from build123d import *
from build123d.topology import SkipClean

# Parameters (mm, degrees)
SKETCH1_R           = 18.161
BOSS_EXTRUDE1_DEPTH = 1.651
BOSS_EXTRUDE2_DEPTH = 5.8928
CUT_EXTRUDE1_REACH  = 45.689
SKETCH5_R           = 13.462
BOSS_EXTRUDE3_DEPTH = 13.335
SKETCH6_R           = 13.462
BOSS_EXTRUDE4_DEPTH = 9.652
BOSS_EXTRUDE4_TAPER = 4
SKETCH7_R           = 13.462
BOSS_EXTRUDE5_DEPTH = 15.24
SKETCH8_R           = 9.398
CUT_EXTRUDE3_DEPTH  = 63.427016824


with BuildPart() as part:
    # Sketch1 → Boss-Extrude1 (new body)
    with BuildSketch(Plane(origin=(0, 0, 0), x_dir=(1, 0, 0), z_dir=(0, 1, 0))):
        with Locations(Location((-14.328841802, 9.162551515, 0), (0, 0, 90))):
            Circle(SKETCH1_R)
    extrude(amount=BOSS_EXTRUDE1_DEPTH)

    # Sketch2 → Boss-Extrude2 (add)
    with BuildSketch(Plane(origin=(0, 1.651, 0), x_dir=(1, 0, 0), z_dir=(0, 1, 0))):
        Polygon((2.466775283, 0.14327327), (1.879890825, 19.198343461), (-14.91572626, 28.217621706), (-31.124458887, 18.18182976), (-30.537574428, -0.87324043), (-13.741957343, -9.892518675), align=None)
    extrude(amount=BOSS_EXTRUDE2_DEPTH)

    # Sketch3 → Cut-Extrude1 (cut, up to next)
    with BuildSketch(Plane(origin=(0, 7.5438, 0), x_dir=(1, 0, 0), z_dir=(0, 1, 0)), mode=Mode.PRIVATE) as cut_extrude1_sk1:
        with BuildLine():
            Line((-13.183471606, 27.287397669), (-14.91572626, 28.217621706))
            Line((-14.91572626, 28.217621706), (-16.587451234, 27.182557187))
            ThreePointArc((-16.587451234, 27.182557187), (-14.887924337, 27.314943857), (-13.183471606, 27.287397669))
        make_face()
    cut_extrude1_tool1 = extrude(cut_extrude1_sk1.sketch, amount=-CUT_EXTRUDE1_REACH, mode=Mode.PRIVATE) & part.part
    # Sketch3 → Cut-Extrude1 (cut, up to next)
    with BuildSketch(Plane(origin=(0, 7.5438, 0), x_dir=(1, 0, 0), z_dir=(0, 1, 0)), mode=Mode.PRIVATE) as cut_extrude1_sk2:
        with BuildLine():
            Line((1.879890825, 19.198343461), (0.147636171, 20.128567497))
            ThreePointArc((0.147636171, 20.128567497), (1.112049838, 18.722927364), (1.940420505, 17.233054906))
            Line((1.940420505, 17.233054906), (1.879890825, 19.198343461))
        make_face()
    cut_extrude1_tool2 = extrude(cut_extrude1_sk2.sketch, amount=-CUT_EXTRUDE1_REACH, mode=Mode.PRIVATE) & part.part
    # Sketch3 → Cut-Extrude1 (cut, up to next)
    with BuildSketch(Plane(origin=(0, 7.5438, 0), x_dir=(1, 0, 0), z_dir=(0, 1, 0)), mode=Mode.PRIVATE) as cut_extrude1_sk3:
        with BuildLine():
            Line((-31.124458887, 18.18182976), (-31.063929206, 16.216541206))
            ThreePointArc((-31.063929206, 16.216541206), (-30.328815977, 17.754568007), (-29.452733913, 19.216894278))
            Line((-29.452733913, 19.216894278), (-31.124458887, 18.18182976))
        make_face()
    cut_extrude1_tool3 = extrude(cut_extrude1_sk3.sketch, amount=-CUT_EXTRUDE1_REACH, mode=Mode.PRIVATE) & part.part
    # Sketch3 → Cut-Extrude1 (cut, up to next)
    with BuildSketch(Plane(origin=(0, 7.5438, 0), x_dir=(1, 0, 0), z_dir=(0, 1, 0)), mode=Mode.PRIVATE) as cut_extrude1_sk4:
        with BuildLine():
            Line((-30.537574428, -0.87324043), (-28.805319774, -1.803464467))
            ThreePointArc((-28.805319774, -1.803464467), (-29.769733441, -0.397824334), (-30.598104109, 1.092048124))
            Line((-30.598104109, 1.092048124), (-30.537574428, -0.87324043))
        make_face()
    cut_extrude1_tool4 = extrude(cut_extrude1_sk4.sketch, amount=-CUT_EXTRUDE1_REACH, mode=Mode.PRIVATE) & part.part
    # Sketch3 → Cut-Extrude1 (cut, up to next)
    with BuildSketch(Plane(origin=(0, 7.5438, 0), x_dir=(1, 0, 0), z_dir=(0, 1, 0)), mode=Mode.PRIVATE) as cut_extrude1_sk5:
        with BuildLine():
            Line((-13.741957343, -9.892518675), (-12.070232369, -8.857454157))
            ThreePointArc((-12.070232369, -8.857454157), (-13.769759266, -8.989840826), (-15.474211997, -8.962294639))
            Line((-15.474211997, -8.962294639), (-13.741957343, -9.892518675))
        make_face()
    cut_extrude1_tool5 = extrude(cut_extrude1_sk5.sketch, amount=-CUT_EXTRUDE1_REACH, mode=Mode.PRIVATE) & part.part
    # Sketch3 → Cut-Extrude1 (cut, up to next)
    with BuildSketch(Plane(origin=(0, 7.5438, 0), x_dir=(1, 0, 0), z_dir=(0, 1, 0)), mode=Mode.PRIVATE) as cut_extrude1_sk6:
        with BuildLine():
            Line((2.466775283, 0.14327327), (2.406245603, 2.108561825))
            ThreePointArc((2.406245603, 2.108561825), (1.671132373, 0.570535023), (0.79505031, -0.891791248))
            Line((0.79505031, -0.891791248), (2.466775283, 0.14327327))
        make_face()
    cut_extrude1_tool6 = extrude(cut_extrude1_sk6.sketch, amount=-CUT_EXTRUDE1_REACH, mode=Mode.PRIVATE) & part.part
    add(cut_extrude1_tool1.solids().sort_by_distance((-14.896658, 7.5438, -27.598516))[0], mode=Mode.SUBTRACT)
    add(cut_extrude1_tool2.solids().sort_by_distance((1.353263, 7.5438, -18.872277))[0], mode=Mode.SUBTRACT)
    add(cut_extrude1_tool3.solids().sort_by_distance((-30.578763, 7.5438, -17.88879))[0], mode=Mode.SUBTRACT)
    add(cut_extrude1_tool4.solids().sort_by_distance((-30.010947, 7.5438, 0.547174))[0], mode=Mode.SUBTRACT)
    add(cut_extrude1_tool5.solids().sort_by_distance((-13.761025, 7.5438, 9.273413))[0], mode=Mode.SUBTRACT)
    add(cut_extrude1_tool6.solids().sort_by_distance((1.92108, 7.5438, -0.436313))[0], mode=Mode.SUBTRACT)

    # Sketch5 → Boss-Extrude3 (add)
    with SkipClean():  # the faces are left unmerged after this step: merging them gives an invalid solid
        with BuildSketch(Plane(origin=(0, 7.5438, 0), x_dir=(1, 0, 0), z_dir=(0, 1, 0))):
            with Locations(Location((-14.273901773, 9.073818285, 0), (0, 0, 270))):
                Circle(SKETCH5_R)
        extrude(amount=BOSS_EXTRUDE3_DEPTH)

    # Sketch6 → Boss-Extrude4 (add)
    with SkipClean():  # the faces are left unmerged after this step: merging them gives an invalid solid
        with BuildSketch(Plane(origin=(0, 20.8788, 0), x_dir=(1, 0, 0), z_dir=(0, 1, 0))):
            with Locations(Location((-14.273901773, 9.073818285, 0), (0, 0, 270))):
                Circle(SKETCH6_R)
        extrude(amount=BOSS_EXTRUDE4_DEPTH, taper=BOSS_EXTRUDE4_TAPER)

    # Sketch7 → Boss-Extrude5 (add)
    with SkipClean():  # the faces are left unmerged after this step: merging them gives an invalid solid
        with BuildSketch(Plane.XZ):
            with Locations(Location((-14.33942015, -8.950735224, 0), (0, 0, 90))):
                Circle(SKETCH7_R)
        extrude(amount=BOSS_EXTRUDE5_DEPTH)

    # Sketch8 → Cut-Extrude3 (cut, through all)
    with SkipClean():  # the faces are left unmerged after this step: merging them gives an invalid solid
        with BuildSketch(Plane.XZ.offset(15.24)):
            with Locations(Location((-14.33942015, -8.950735224, 0), (0, 0, 270))):
                Circle(SKETCH8_R)
        extrude(amount=-CUT_EXTRUDE3_DEPTH, mode=Mode.SUBTRACT)


solid = part.part
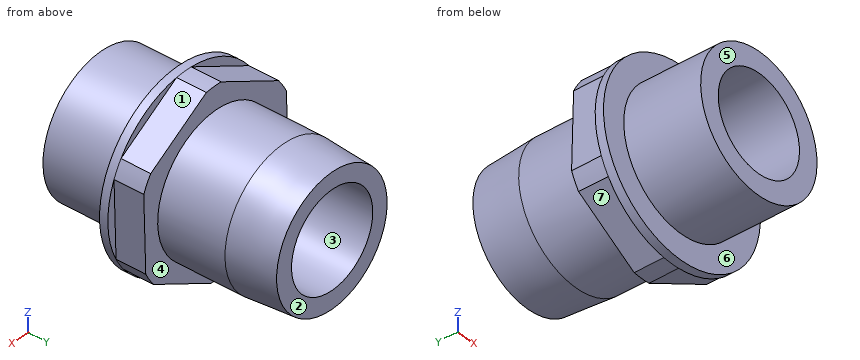
The listing builds one solid part. Answer for the finished solid, in the listing's coordinates (mm). Face numbers are marked on the shaded views. A direction names the side the tool comes from. Coordinates: 2 decimals unless noted, no trailing zeros. Order: outer loops, then holes, each group sorted by start corner. A loop starts at its lowest first (then second) coordinate and runs counter-clockwise, first axis right, second up.
Q1. Consider line 1 (Z direction, x = -14.5, y = 17); line 2 (Y direction, x = -5.5, z = -24); line 3 (X direction, y = 8, z = -13.5). Determine where each line is inside the solid, lowest interval first.
Q2. A cutting plane is placed at C-C, the plane y = 26. Write down the section's boundary in (x, z).
Q3. For a pull along Z with two mould halves and no side action, classify the marked faces 1, 2 and 3 as pulls with the +Z half, pulls with the -Z half, needs draft (parallel to the pull), parting line crosses it, or undercut.
Q4. Which of the six approach directions +Z, -Z, +X, -X, +Y, -Y give full straight-line access (tool end or side, diameter ignored) to the marked faces 4, 5, 6 and 7?
Q5. A cutting plane is placed at D-D, the plane y = 17. Write down the section's boundary in (x, z), and give its area (3 significant figures).
Q6. A cutting plane is placed at A-A, the plane y = 6. Write down the section's boundary in (x, z), and give its area (3 significant figures).
Q7. A cutting plane is placed at B-B, the plane z = 5.5. Write down the section's boundary in (x, y), and give its area (3 significant figures).
Q8. Given P1, Ø10, axis at x = -12.5, z = -11.5, coming from the +Y side; P2, Ø0.9, axis at x = 3, z = -8.5, coming from the +Y side; P3, Ø6.5, axis at x = -25.5, z = -22.5, coming from the +Y side; P4, Ø8, axis at x = -16, y = 16.5, coming from the +Z side, each flat-ended and moving along its own axis, determine where each tip first touches the part or whether it passes through.
Answers follow:
1. line 1: z = -22.53 to -18.35, 0.45 to 4.39
1. line 2: y = 0 to 1.65
1. line 3: x = -26.99 to -22.56, -6.12 to -1.56
2. outline: circle Ø26.21 at (-14.27, -9.07); hole circle Ø18.8 at (-14.34, -8.95)
3. face 1: pulls with the +Z half
3. face 2: needs draft
3. face 3: undercut
4. face 4: +Y
4. face 5: +Z, -Z, +X, -X, -Y
4. face 6: -Y
4. face 7: -Z, -X, +Y
5. outline: circle Ø26.92 at (-14.27, -9.07); hole circle Ø18.8 at (-14.34, -8.95)
5. area: 292 mm2
6. outline: (-31.06, -16.22) arc R18.16 ccw to (-29.45, -19.22) - (-16.59, -27.18) arc R18.16 ccw to (-13.18, -27.29) - (0.15, -20.13) arc R18.16 ccw to (1.94, -17.23) - (2.41, -2.11) arc R18.16 ccw to (0.8, 0.89) - (-12.07, 8.86) arc R18.16 ccw to (-15.47, 8.96) - (-28.81, 1.8) arc R18.16 ccw to (-30.6, -1.09) - close; hole circle Ø18.8 at (-14.34, -8.95)
6. area: 658 mm2
7. outline: (-25.04, 0) - (-3.61, 0) - (-3.61, 1.65) - (-6.65, 1.65) - (-6.65, 7.54) - (-21.92, 7.54) - (-21.92, 1.65) - (-25.04, 1.65) - close
7. area: 125 mm2
8. P1: passes through
8. P2: stops at y = 1.65
8. P3: stops at y = 7.54
8. P4: stops at z = 4.39
